```python
from build123d import *

# Parameters (mm, degrees)
SWEEP1_PROFILE_R     = 6.35
CUT_SWEEP1_PROFILE_R = 3.175


with BuildPart() as part:
    # Sweep1: sweep along a curve in space
    with BuildLine() as sweep1_path:
        Line((44.09223227, 18.666797388, 9.772665845), (44.09223227, 18.666797388, -12.977334155))
        ThreePointArc((44.09223227, 18.666797388, 9.772665845), (83.44709616, 47.763643929, 75.881872817), (145.777808921, 93.847583872, 48.36802607))
        ThreePointArc((145.777808921, 93.847583872, 48.36802607), (186.971547467, 138.178197356, -19.900895831), (224.914532295, 206.184188109, -67.422345819))
        ThreePointArc((233.124989376, 243.66897146, -75.320122751), (230.785950694, 224.145501617, -73.242307626), (224.914532295, 206.184188109, -67.422345819))
        Line((233.347766263, 252.639211932, -75.379620636), (233.124989376, 243.66897146, -75.320122751))
        Line((233.823290134, 271.786456188, -75.506620636), (233.347766263, 252.639211932, -75.379620636))
    # Sweep1 profile (on start of the path) → Sweep1 (sweep)
    with BuildSketch(Plane(origin=(233.823290134, 271.786456188, -75.506620636), x_dir=(-0.999691751300367, 0.024827452185136066, 0), z_dir=(-0.02482690640849771, -0.9996697752877118, 0.006630617950041174))):
        Circle(SWEEP1_PROFILE_R)
    sweep(path=sweep1_path.line)

    # Cut-Sweep1: sweep along a curve in space
    with BuildLine() as cut_sweep1_path:
        Line((44.09223227, 18.666797388, 9.772665845), (44.09223227, 18.666797388, -12.977334155))
        ThreePointArc((44.09223227, 18.666797388, 9.772665845), (83.44709616, 47.763643929, 75.881872817), (145.777808921, 93.847583872, 48.36802607))
        ThreePointArc((145.777808921, 93.847583872, 48.36802607), (186.971547467, 138.178197356, -19.900895831), (224.914532295, 206.184188109, -67.422345819))
        ThreePointArc((233.124989376, 243.66897146, -75.320122751), (230.785950694, 224.145501617, -73.242307626), (224.914532295, 206.184188109, -67.422345819))
        Line((233.347766263, 252.639211932, -75.379620636), (233.124989376, 243.66897146, -75.320122751))
        Line((233.823290134, 271.786456188, -75.506620636), (233.347766263, 252.639211932, -75.379620636))
    # Cut-Sweep1 profile (on start of the path) → Cut-Sweep1 (sweep, cut)
    with BuildSketch(Plane(origin=(233.823290134, 271.786456188, -75.506620636), x_dir=(-0.999691751300367, 0.024827452185136066, 0), z_dir=(-0.02482690640849771, -0.9996697752877118, 0.006630617950041174))):
        Circle(CUT_SWEEP1_PROFILE_R)
    sweep(path=cut_sweep1_path.line, mode=Mode.SUBTRACT)


solid = part.part
```
The model under review builds one solid part; all positions refer to its coordinate system, in mm. Round coordinates to 2 decimals unless told otherwise and drop trailing zeros. Use a Markdown table: item, result. Add a question column.
Q1. The part is to be moulded in two halves that separate along Y. For faces 1 (the face through (47, 17, -12.977)), 2 (the face through (37.967, 20.34, -1.762)), 3 (the face through (41.208, 17.339, -1.762)), say which applies: pulls with the +Y half, pulls with the -Y half, needs draft (parallel to the pull), parting line crosses it, or undercut.
Q2. Add section A-A (z = 65.5). State how many separate pieces and enclosed holes the cut face has, plus the area to 3 significant figures.
Q3. Insertion check: pin 1 Ø8 at (x, z) = (134, 58.5) entering from +Y; pin 2 Ø12 at (y, z) = (158.5, -39.5) entering from -X; pin 3 Ø6.5 at (x, y) = (43, 18.5) entering from -Z. Each pin has a flat end and moves straight along its axis. Give the tip position at first contact, or say it passes through.
Q4. For probe 1 along Z at (x, y) = (99, 55), list the stretches that pass through material, from the lowest coordinate up.
Worked answers:
| question | item | result |
|---|---|---|
| 1 | face 1 | needs draft |
| 1 | face 2 | parting line crosses it |
| 1 | face 3 | undercut |
| 2 | separate pieces | 2 |
| 2 | enclosed holes | 2 |
| 2 | area | 329 mm² |
| 3 | pin 1 | y = 95.68 |
| 3 | pin 2 | x = 190.68 |
| 3 | pin 3 | z = -12.98 |
| 4 | probe 1 | 73.46 to 84.16 |
